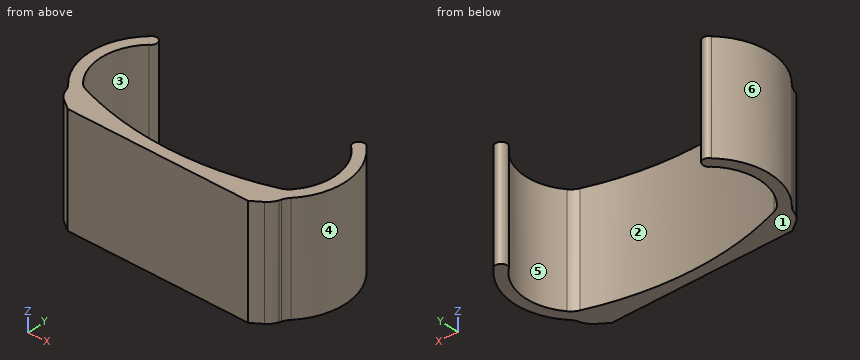
from build123d import *

# Parameters (mm, degrees)
F1_DEPTH = 30
F2_SIZE  = 3
F3_R     = 5


with BuildPart() as f1:
    # F0 (on Top) → F1 (new body)
    with BuildSketch(Plane.XY):
        with BuildLine():
            Line((-29.235905425, 4.8452048085), (-27.5, 0))
            Line((-27.5, 0), (27.5, 0))
            Line((27.5, 0), (29.235905425, 4.8452048085))
            ThreePointArc((29.235905425, 4.8452048085), (29.6607503771, 5.7400765845), (30.2536774297, 6.533629506))
            ThreePointArc((30.2536774297, 6.533629506), (34.7005588033, 18.4719723629), (29.5974730182, 30.1449025686))
            ThreePointArc((29.5974730182, 30.1449025686), (27.0806665873, 30.5080582414), (27.5, 28))
            ThreePointArc((27.5, 28), (31.6871939258, 18.746306096), (28.5098241443, 9.0991425174))
            ThreePointArc((28.5098241443, 9.0991425174), (27.527116318, 8.1895587275), (26.3382475055, 7.5734026682))
            ThreePointArc((26.3382475055, 7.5734026682), (0.0002388204, 3.0000000025), (-26.337843619, 7.5729779002))
            ThreePointArc((-26.337843619, 7.5729779002), (-27.5266380589, 8.1890555536), (-28.5093137303, 9.0985237608))
            ThreePointArc((-28.5093137303, 9.0985237608), (-31.6872153169, 18.7459056114), (-27.5, 28))
            ThreePointArc((-27.5, 28), (-27.0806665873, 30.5080582414), (-29.5974730182, 30.1449025686))
            ThreePointArc((-29.5974730182, 30.1449025686), (-34.7005588033, 18.4719723629), (-30.2536774297, 6.533629506))
            ThreePointArc((-30.2536774297, 6.533629506), (-29.6607503771, 5.7400765845), (-29.235905425, 4.8452048085))
        make_face()
    extrude(amount=F1_DEPTH)

    # F2
    f2_edges = [f1.edges().sort_by_distance(p)[0] for p in [
        (-27.5, 0, 15),
        (27.5, 0, 15),
    ]]
    chamfer(f2_edges, length=F2_SIZE)

    # F3
    f3_edges = [f1.edges().sort_by_distance(p)[0] for p in [
        (-28.511839, 2.824213, 15),
        (28.511839, 2.824213, 15),
    ]]
    fillet(f3_edges, radius=F3_R)


solid = f1.part
For this review, take the finished solid that the model builds, in its own axes (mm). Face numbers are marked on the shaded views. A direction names the side the tool comes from. Give positions to 0.01 mm unless a question says otherwise; leave off trailing zeros. Loops run counter-clockwise (first coordinate to the right, second up) from the corner with the lowest first, then second, coordinate; pieces in that order, holes last.
Item 1: Take a section at C-C, the plane y = 10.5. State the section outline as (x, z) points.
Item 2: Take a section at D-D, the plane x = -14.5. State the section outline as (y, z) points, and give its area (3 significant figures).
Item 3: For line 1 along X through (y, z) = (15, 3.5); line 2 along X through (y, z) = (12, 14.25); line 3 along Y through (x, z) = (30, 10), list the stretches that pass through material, from the lowest coordinate up.
Item 4: Insertion check: pin 1 (10 mm diameter, centred on y = 4.5, z = 22.5, fed in from +X); pin 2 (1.5 mm diameter, centred on y = 20.5, z = 8, fed in from +X); pin 3 (4 mm diameter, centred on y = 4, z = 15.5, fed in from +X). Each pin has a flat end and moves straight along its axis. Give the tip position at first contact, or say it passes through.
Item 5: Take a section at B-B, the plane z = 12.5. State the section outline as (x, y) points.
Item 6: Take a section at A-A, the plane y = 14.5. State the section outline as (x, z) points, and give its area (3 significant figures).
Item 7: Tool access review of the marked faces 5 and 6: name each direction out of +Z, -Z, +X, -X, +Y, -Y from which nothing blocks a thin tool from reaching the whole face with its end or side.
Item 8: Draft analysis for pull direction X (two halves, no side actions). For the marked faces 1, 2, 3 and 4, state which applies: +X half, -X half, draft (parallel to the pull), parting line (faces both ways), or undercut.
Calculated:
1. outline: (-32.96, 0) - (-29.53, 0) - (-29.53, 30) - (-32.96, 30) - close; (29.53, 0) - (32.96, 0) - (32.96, 30) - (29.53, 30) - close
2. outline: (0, 0) - (4.36, 0) - (4.36, 30) - (0, 30) - close
2. area: 131 mm2
3. line 1: x = -34.44 to -31.38, 31.38 to 34.44
3. line 2: x = -33.61 to -30.35, 30.35 to 33.61
3. line 3: y = 6.23 to 11.3, 24.7 to 29.74
4. pin 1: stops at x = 32.43
4. pin 2: stops at x = 34.62
4. pin 3: stops at x = 29.83
5. outline: (-30.25, 6.53) arc R5 cw to (-29.24, 4.85) - (-29.05, 4.31) arc R5 ccw to (-27.22, 1.91) - (-24.5, 0) - (24.5, 0) - (27.22, 1.91) arc R5 ccw to (29.05, 4.31) - (29.24, 4.85) arc R5 cw to (30.25, 6.53) arc R16.99 ccw to (29.6, 30.14) arc R1.57 ccw (long way) to (27.5, 28) arc R13.99 cw to (28.51, 9.1) arc R5 cw to (26.34, 7.57) arc R78.13 cw to (-26.34, 7.57) arc R5 cw to (-28.51, 9.1) arc R13.99 cw to (-27.5, 28) arc R1.57 ccw (long way) to (-29.6, 30.14) arc R16.99 ccw to start
6. outline: (-34.34, 0) - (-31.26, 0) - (-31.26, 30) - (-34.34, 30) - close; (31.26, 0) - (34.34, 0) - (34.34, 30) - (31.26, 30) - close
6. area: 185 mm2
7. face 5: +Z, -Z
7. face 6: +Z, -Z, -X
8. face 1: draft
8. face 2: undercut
8. face 3: undercut
8. face 4: +X half
